Autodesk Fusion 360 part; units mm, degrees
box "BoxPrimitive1" add length 90 width 100 height 2 placed x (0, 0, 1) y (1, 0, 0) z (0, 1, 0) at (0, 0, -10)
box "BoxPrimitive2" cut length 20 width 28 height -10 placed x (0, 0, -1) y (-1, 0, 0) z (0, 1, 0) at (64, 2, 40)
box "BoxPrimitive3" cut length 5 width 28 height -1 placed x (0, 0, -1) y (-1, 0, 0) z (0, 1, 0) at (64, 2, 20)
Model file for the job. Use its own axes, mm. Give positions to 0.01 mm unless a question says otherwise; leave off trailing zeros. Order: outer loops, then holes, each group sorted by start corner. A loop starts at its lowest first (then second) coordinate and runs counter-clockwise, first axis right, second up. Notation, with made-up numbers: (-21.75, 49) - (-16.75, 49) arc R16 ccw to (-16.75, 63) - close; hole circle Ø1 at (17.5, 70.25). An arc over 180 degrees is marked (long way). Write item = value, one per line. Start each with the question number.
1. Cut at A-A, the plane z = 25.5. List the corners of the cut face in (x, y), and give its area (3 significant figures).
2. Two-plate mould, pull along X, no slides. Class faces 1 (the flat face through (50, 1, 18)), 2 (the flat face through (51, 0, 44)): pulls with the +X half, pulls with the -X half, needs draft (parallel to the pull), parting line crosses it, or undercut.
3. Cut at B-B, the plane x = 37.5. List the corners of the cut face in (y, z), and give its area (3 significant figures).
4. Cut at C-C, the plane y = 0.6. List the corners of the cut face in (x, z), and give its area (3 significant figures).
5. Probe line 1 along X through (y, z) = (0.6, 27); line 2 along Z through (x, y) = (45, 1.5); line 3 along Z through (x, y) = (59, 0.35). List the from-to ranges inside material, lowest first.
6. Drop flat-ended pins along their axis: P1, Ø4, axis at x = 50.5, z = 17.5, coming from the +Y side; P2, Ø2, axis at x = 11, z = 33, coming from the -Y side. Give the stop position or say it passes through.
Taken from the geometry:
q1.outline = (0, 0) - (36, 0) - (36, 2) - (0, 2) - close; (64, 0) - (100, 0) - (100, 2) - (64, 2) - close
q1.area = 144 mm²
q2.face_1 = undercut
q2.face_2 = needs draft
q3.outline = (0, -10) - (2, -10) - (2, 15) - (1, 15) - (1, 20) - (0, 20) - close; (0, 40) - (2, 40) - (2, 80) - (0, 80) - close
q3.area = 135 mm²
q4.outline = (0, -10) - (100, -10) - (100, 80) - (0, 80) - close; hole (36, 20) - (64, 20) - (64, 40) - (36, 40) - close
q4.area = 8,440 mm²
q5.line_1 = 0 to 36, 64 to 100
q5.line_2 = -10 to 15, 40 to 80
q5.line_3 = -10 to 20, 40 to 80
q6.P1 = 1
q6.P2 = 0
